Design review of the part built by this model. Coordinates are the model's own, in mm. A direction names the side the tool comes from. Coordinates: 2 decimals unless noted, no trailing zeros. Order: outer loops, then holes, each group sorted by start corner. A loop starts at its lowest first (then second) coordinate and runs counter-clockwise, first axis right, second up. Notation, with made-up numbers: M 53,49 L 70,49 A27 ccw 70,72 Z; hole C 14,-1 d10. An arc over 180 degrees is marked long. Answer as a JSON object with one key per item and string values.
from build123d import *

# Parameters (mm, degrees)
SKETCH1_R           = 63.5
BOSS_EXTRUDE1_DEPTH = 50.8
SKETCH2_R           = 60.325
SKETCH2_R_2         = 57.15
BOSS_EXTRUDE2_DEPTH = 6.35
SKETCH3_R           = 60.325
CUT_EXTRUDE1_DEPTH  = 53.975
CUT_EXTRUDE1_DRAFT  = -5
SKETCH4_R           = 4.7625
CUT_EXTRUDE3_DEPTH  = 3.175


with BuildPart() as part:
    # Sketch1 → Boss-Extrude1 (new body)
    with BuildSketch(Plane(origin=(0, 0, 0), x_dir=(1, 0, 0), z_dir=(0, 1, 0))):
        with Locations(Location((0, 0, 0), (0, 0, 270))):
            Circle(SKETCH1_R)
    extrude(amount=BOSS_EXTRUDE1_DEPTH)

    # Sketch2 → Boss-Extrude2 (add)
    with BuildSketch(Plane.XZ):
        with Locations(Location((0, 0, 0), (0, 0, 270))):
            Circle(SKETCH2_R)
        Circle(SKETCH2_R_2, mode=Mode.SUBTRACT)
        Circle(SKETCH2_R_2)
    extrude(amount=BOSS_EXTRUDE2_DEPTH)


with BuildPart() as cut_extrude1_tool:
    # Sketch3 → Cut-Extrude1 (with draft: the straight prism first)
    with BuildSketch(Plane(origin=(0, 50.8, 0), x_dir=(1, 0, 0), z_dir=(0, 1, 0))):
        with Locations(Location((0, 0, 0), (0, 0, 90))):
            Circle(SKETCH3_R)
    extrude(amount=-CUT_EXTRUDE1_DEPTH)
    # Cut-Extrude1: the draft: its side faces are tilted about the plane it starts from
    cut_extrude1_sides = [cut_extrude1_tool.faces().sort_by_distance(p)[0] for p in [
        (0, 23.8125, 60.325),
    ]]
    draft(cut_extrude1_sides, Plane(origin=(0, 50.8, 0), x_dir=(1, 0, 0), z_dir=(0, 1, 0)), CUT_EXTRUDE1_DRAFT)


with BuildPart() as part_1:
    add(part.part)

    # Cut-Extrude1: cut by cut_extrude1_tool
    add(cut_extrude1_tool.part, mode=Mode.SUBTRACT)

    # Sketch4 → Cut-Extrude3 (cut)
    with BuildSketch(Plane(origin=(0, -3.175, 0), x_dir=(1, 0, 0), z_dir=(0, 1, 0))):
        with Locations(Location((7.487131795, -15.775986934, 0), (0, 0, 270))):
            Circle(SKETCH4_R)
        with Locations(Location((0, 0, 0), (0, 0, 270))):
            Circle(SKETCH4_R)
        with Locations(Location((-7.487131795, 15.775986934, 0), (0, 0, 270))):
            Circle(SKETCH4_R)
    extrude(amount=-CUT_EXTRUDE3_DEPTH, mode=Mode.SUBTRACT)


solid = part_1.part
1) Insertion check: pin 1 Ø4 at (y, z) = (7, 0) entering from -X; pin 2 Ø5 at (x, y) = (4, 3) entering from -Z; pin 3 Ø12.5 at (x, z) = (-7.49, -15.78) entering from -Y; pin 4 Ø5 at (x, y) = (-37.5, 25) entering from +Z. Each pin has a flat end and moves straight along its axis. Give the tip position at first contact, or say it passes through.
Taken from the geometry:
{"pin 1": "stops at x = -63.5", "pin 2": "stops at z = -63.48", "pin 3": "stops at y = -6.35", "pin 4": "stops at z = 52.98"}
2) To check wall thickness, follow L1, parallel to X at y = -4, z = 0 (1 decimal); L2, parallel to Y at x = 38.5, z = -25 (3 decimals); L3, parallel to X at y = 13, z = 26.5. State the ranges of each line that lie inside material, in increasing order.
Taken from the geometry:
{"L1": "x = -60.3 to -4.8, 4.8 to 60.3", "L2": "y = -6.35 to -3.175", "L3": "x = -57.71 to -50.49, 50.49 to 57.71"}
3) Add section C-C (y = 22). State the section outline as (x, z) points.
Taken from the geometry:
{"outline": "C 0,0 d127; hole C 0,0 d115.61"}
4) Tool access review of faces 4 (the cylindrical face through (-61.99, 25.04, -13.77)), 5 (the flat face through (12, -3.175, 1)), 6 (the flat face through (-23, 0, 56)): name each direction out of +Z, -Z, +X, -X, +Y, -Y from which nothing blocks a thin tool from reaching the whole face with its end or side.
Taken from the geometry:
{"face 4": "+Y, -Y", "face 5": "+Y", "face 6": "-Y"}
5) Mouldability with a two-part tool opening along Z and no side actions: class faces 1 (the cylindrical face through (-7.278, -4.74, -20.534)), 2 (the flat face through (-23, 50.8, 56)), 3 (the cylindrical face through (2.652, -3.131, 60.267)) as released by +Z, released by -Z, zero draft, split by the parting line, or undercut.
Taken from the geometry:
{"face 1": "undercut", "face 2": "zero draft", "face 3": "split by the parting line"}
6) Add section D-D (y = 2). State the section outline as (x, z) points.
Taken from the geometry:
{"outline": "C 0,0 d127; hole C 0,0 d112.11"}
